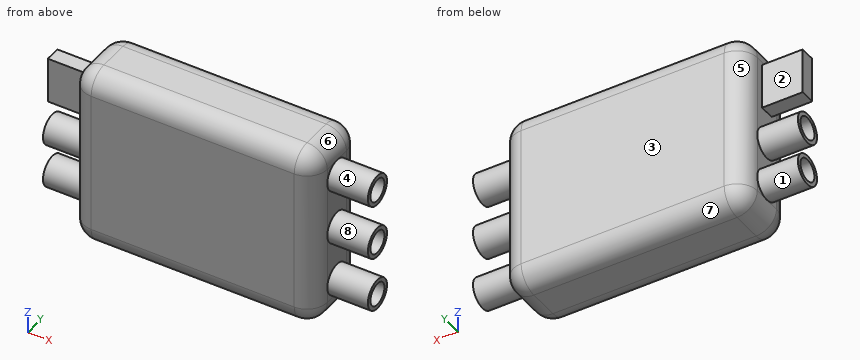
from build123d import *

# Parameters (mm, degrees)
BOSS_EXTRUDE1_DEPTH = 7
FILLET1_R           = 2
SKETCH2_R           = 1.5
SKETCH2_R_2         = 1.1
BOSS_EXTRUDE2_DEPTH = 4
SKETCH3_R           = 1.5
SKETCH3_R_2         = 1.1
SKETCH3_W           = 4.5
SKETCH3_H           = 1.5
BOSS_EXTRUDE3_DEPTH = 4


with BuildPart() as part:
    # Sketch1 → Boss-Extrude1 (new body)
    with BuildSketch(Plane(origin=(0, 0, 0), x_dir=(1, 0, 0), z_dir=(0, 1, 0))):
        with BuildLine():
            Line((10, -9), (-10, -9))
            ThreePointArc((-10, -9), (-11.414213562, -8.414213562), (-12, -7))
            Line((-12, -7), (-12, 7))
            ThreePointArc((-12, 7), (-11.414213562, 8.414213562), (-10, 9))
            Line((-10, 9), (10, 9))
            ThreePointArc((10, 9), (11.414213562, 8.414213562), (12, 7))
            Line((12, 7), (12, -7))
            ThreePointArc((12, -7), (11.414213562, -8.414213562), (10, -9))
        make_face()
    extrude(amount=BOSS_EXTRUDE1_DEPTH)

    # Fillet1
    fillet1_edges = [part.edges().sort_by_distance(p)[0] for p in [
        (12, 0, 0),
        (11.414213562, 0, 8.414213562),
        (0, 0, 9),
        (-11.414213562, 0, 8.414213562),
        (11.414213562, 7, 8.414213562),
        (12, 7, 0),
        (11.414213562, 7, -8.414213562),
        (0, 7, -9),
        (-11.414213562, 7, -8.414213562),
        (-12, 7, 0),
        (-11.414213562, 7, 8.414213562),
        (-12, 0, 0),
        (0, 7, 9),
        (-11.414213562, 0, -8.414213562),
        (0, 0, -9),
        (11.414213562, 0, -8.414213562),
    ]]
    fillet(fillet1_edges, radius=FILLET1_R)

    # Sketch2 → Boss-Extrude2 (add)
    with BuildSketch(Plane(origin=(12, 0, 0), x_dir=(0, 0, -1), z_dir=(1, 0, 0))):
        with Locations((0, 3.5)):
            Circle(SKETCH2_R)
        with Locations((0, 3.5)):
            Circle(SKETCH2_R_2, mode=Mode.SUBTRACT)
        with Locations((-5.476648667, 3.5)):
            Circle(SKETCH2_R)
        with Locations((-5.476648667, 3.5)):
            Circle(SKETCH2_R_2, mode=Mode.SUBTRACT)
        with Locations((5.464786958, 3.5)):
            Circle(SKETCH2_R)
        with Locations((5.464786958, 3.5)):
            Circle(SKETCH2_R_2, mode=Mode.SUBTRACT)
    extrude(amount=BOSS_EXTRUDE2_DEPTH)

    # Sketch3 → Boss-Extrude3 (add)
    with BuildSketch(Plane.ZY.offset(12)):
        with Locations((-1.091059361, 3.5)):
            Circle(SKETCH3_R)
        with Locations((-1.091059361, 3.5)):
            Circle(SKETCH3_R_2, mode=Mode.SUBTRACT)
        with Locations((-5.491059361, 3.5)):
            Circle(SKETCH3_R)
        with Locations((-5.491059361, 3.5)):
            Circle(SKETCH3_R_2, mode=Mode.SUBTRACT)
        with Locations((4.47030055, 3.5)):
            Rectangle(SKETCH3_W, SKETCH3_H)
    extrude(amount=BOSS_EXTRUDE3_DEPTH)


solid = part.part
Input: part model. Units: mm. Frame: model coordinates. Face numbers are marked on the shaded views. A direction names the side the tool comes from. Coordinates: 2 decimals unless noted, no trailing zeros. Order: outer loops, then holes, each group sorted by start corner. A loop starts at its lowest first (then second) coordinate and runs counter-clockwise, first axis right, second up. Notation, with made-up numbers: M -29.5,-31 L 4.5,-31 A11 ccw 4.5,-24 Z; hole C 12,-6 d11. An arc over 180 degrees is marked long. Write item = value, one per line. Start each with the question number.
(1) Line query: line 1 along Z through (x, y) = (14, 4.5); line 2 along X through (y, z) = (3.5, -0.75); line 3 along Z through (x, y) = (-2.5, 0.75). Output: solid intervals per line, ascending. Write a range as [from, to].
(2) Reachability of the marked faces 1, 2, 3, 4 and 5 from +Z, -Z, +X, -X, +Y, -Y: full face, straight path, thin tool, end or side. Return the list, or none.
(3) Section D-D on z = 6.25. Output: boundary loops of the cut face in (x, y), and give its area (3 significant figures).
(4) Pull-direction query (Z, two-part tool) for the marked faces 6, 7 and 8; classes: released by +Z, released by -Z, zero draft, split by the parting line, or undercut.
(5) Section C-C on y = 1.25. Output: boundary loops of the cut face in (x, z).
(6) Section B-B on x = -5. Output: boundary loops of the cut face in (y, z), and give its area (3 significant figures).
(7) First-contact query: P1, Ø1.1, axis at y = 4, z = -1.5, coming from the -X side; P2, Ø1.8, axis at y = 3.5, z = -5.49, coming from the -X side; P3, Ø1, axis at y = 3.5, z = -0.5, coming from the +X side; P4, Ø1, axis at x = 10, y = 1, coming from the +Z side. Flat tips, straight axial feed; report the tip coordinate or a pass-through.
(8) Section A-A on x = -12.5. Output: boundary loops of the cut face in (y, z), and give its area (3 significant figures).
Result set:
q1.line_1 = [-6.58, -5.92], [-5.01, -4.35], [-1.12, -0.46], [0.46, 1.12], [4.36, 5.02], [5.93, 6.59]
q1.line_2 = [-12, 12]
q1.line_3 = [-8.56, 8.56]
q2.face_1 = -X
q2.face_2 = +Z, -X, +Y
q2.face_3 = +Z, -Z, +X, -X, +Y
q2.face_4 = +X
q2.face_5 = +Z, -Z, -X, +Y
q3.outline = M -16,2.75 L -12,2.75 L -12,2 A2 ccw -10,0 L 10,0 A2 ccw 12,2 L 12,2.21 L 16,2.21 L 16,2.72 L 12,2.72 L 12,4.28 L 16,4.28 L 16,4.79 L 12,4.79 L 12,5 A2 ccw 10,7 L -10,7 A2 ccw -12,5 L -12,4.25 L -16,4.25 Z
q3.area = 175 mm²
q4.face_6 = released by +Z
q4.face_7 = released by -Z
q4.face_8 = undercut
q5.outline = M -11.85,-7 A1.85 ccw -10,-8.85 L 10,-8.85 A1.85 ccw 11.85,-7 L 11.85,7 A1.85 ccw 10,8.85 L -10,8.85 A1.85 ccw -11.85,7 Z
q6.outline = M 0,-7 A2 ccw 2,-9 L 5,-9 A2 ccw 7,-7 L 7,7 A2 ccw 5,9 L 2,9 A2 ccw 0,7 Z
q6.area = 123 mm²
q7.P1 = -16
q7.P2 = -12
q7.P3 = 12
q7.P4 = 8.94
q8.outline = C 3.5,-5.49 d3; C 3.5,-1.09 d3; M 2.75,2.22 L 4.25,2.22 L 4.25,6.72 L 2.75,6.72 Z; hole C 3.5,-5.49 d2.2; hole C 3.5,-1.09 d2.2
q8.area = 13.3 mm²
